Could you check a few things on this drawing? It's one solid part, dimensions in mm from its lowest x, y, z. A direction names the side the tool comes from. Coordinates: 2 decimals unless noted, no trailing zeros. Order: outer loops, then holes, each group sorted by start corner. A loop starts at its lowest first (then second) coordinate and runs counter-clockwise, first axis right, second up. Notation, with made-up numbers: M 69,43.5 L 104,43.5 A12 ccw 104,64.5 Z; hole C 36.25,22 d10. An arc over 180 degrees is marked long. One line per question, with ' | ' between items. Start each with the question number.
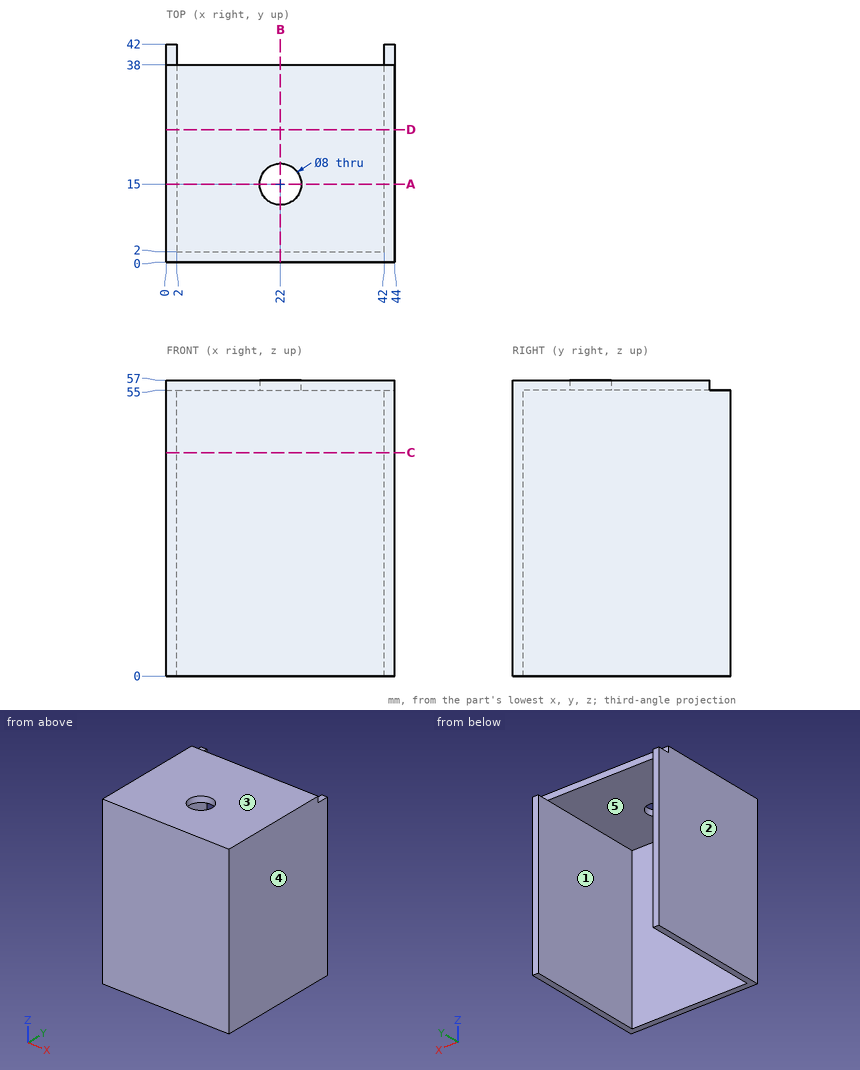
1. Imagine slicing it at C-C (z = 43). List the corners of the cut face in (x, y) for me, then the cut area to 3 significant figures.
2. Imagine slicing it at A-A (y = 15). List the corners of the cut face in (x, z) for me, then the cut area to 3 significant figures.
3. Imagine slicing it at D-D (y = 25.5). List the corners of the cut face in (x, z) for me, then the cut area to 3 significant figures.
4. Imagine slicing it at B-B (x = 22). List the corners of the cut face in (y, z) for me, then the cut area to 3 significant figures.
5. Which directions (+Z, -Z, +X, -X, +Y, -Y) give clear straight access to the entire face, cutting with the end or side of a thin tool? Please do the marked faces 1 and 2.
6. We'd pull the mould along X, two halves only. Please class the marked faces 3, 4 and 5: released by +X, released by -X, zero draft, split by the parting line, or undercut.
7. I need wall thicknesses on line 1 (X direction, y = 9.5, z = 54.5); line 2 (Y direction, x = 22, z = 55.65); line 3 (X direction, y = 15, z = 56). Which ranges of each line are inside material? Lowest first, please.
8. Will these pins go through, and if not, where does the flat tip stop? pin 1 (2 mm diameter, centred on x = 12.5, z = 56, fed in from +Y); pin 2 (18 mm diameter, centred on x = 13, y = 26.5, fed in from -Z); pin 3 (0.6 mm diameter, centred on x = 0.5, y = 40.5, fed in from +Z); pin 4 (6.5 mm diameter, centred on x = 22, y = 15, fed in from +Z).
Entries:
1) outline: M 0,0 L 44,0 L 44,42 L 42,42 L 42,2 L 2,2 L 2,42 L 0,42 Z | area: 248 mm²
2) outline: M 0,0 L 2,0 L 2,55 L 18,55 L 18,57 L 0,57 Z; M 26,55 L 42,55 L 42,0 L 44,0 L 44,57 L 26,57 Z | area: 292 mm²
3) outline: M 0,0 L 2,0 L 2,55 L 42,55 L 42,0 L 44,0 L 44,57 L 0,57 Z | area: 308 mm²
4) outline: M 0,0 L 2,0 L 2,55 L 11,55 L 11,57 L 0,57 Z; M 19,55 L 38,55 L 38,57 L 19,57 Z | area: 170 mm²
5) face 1: -Z, +Y | face 2: +Z, -Z, -X, +Y, -Y
6) face 3: zero draft | face 4: released by +X | face 5: undercut
7) line 1: 0 to 2, 42 to 44 | line 2: 0 to 11, 19 to 38 | line 3: 0 to 18, 26 to 44
8) pin 1: y = 38 | pin 2: z = 55 | pin 3: z = 55 | pin 4: through
